Source: CAD feature listing. Evaluate the final solid. Frame: model axes, mm. A direction names the side the tool comes from. Coordinates: 2 decimals unless noted, no trailing zeros. Order: outer loops, then holes, each group sorted by start corner. A loop starts at its lowest first (then second) coordinate and runs counter-clockwise, first axis right, second up.
Item 1: Ray query, line 1 (X direction, y = 12.5, z = 18.5); line 2 (X direction, y = 3, z = 16); line 3 (Y direction, x = 19, z = 15.5) (3 decimals). Return the intervals inside material, ascending.
Item 2: Section C-C on x = -29.5. Return the cut outline in (y, z) (3 decimals).
Item 3: Section A-A on y = 11. Return the cut outline in (x, z).
Item 4: Section D-D on z = 21.25. Return the cut outline in (x, y) (3 decimals), then the cut area to 3 significant figures.
Item 5: Reachability of faces 1 (the flat face through (-35.306, 16, 13)), 2 (the flat face through (38.481, 18, 13)), 3 (the cylindrical face through (-51.128, 1.565, 19.875)) from +Z, -Z, +X, -X, +Y, -Y: full face, straight path, thin tool, end or side. Return the list, or none.
Item 6: Section B-B on z = 9.25. Return the cut outline in (x, y) (3 decimals), then the cut area to 3 significant figures.
Item 7: Contact query for flat-ended pins moving along their axis: P1, Ø8, axis at y = 15.5, z = 16, coming from the +X side; P2, Ø12.5, axis at x = -9.5, z = 8, coming from the -Y side; P3, Ø2, axis at y = 15, z = 15, coming from the -X side. Output: stop coordinate, or through.
from build123d import *

# Parameters (mm, degrees)
F1_DEPTH = 25.4
F2_R     = 3.175
F4_DEPTH = 32.386
F5_R     = 6.35


with BuildPart() as f1:
    # F0 (on Top) → F1 (new body)
    with BuildSketch(Plane.XY):
        Polygon((-35.306, 29.21), (0, 29.21), (35.306, 29.21), (35.306, 0), (63.881, 0), (63.881, 3.175), (38.481, 3.175), (38.481, 32.385), (0, 32.385), (-38.481, 32.385), (-38.481, 3.175), (-63.881, 3.175), (-63.881, 0), (-35.306, 0), align=None)
    extrude(amount=F1_DEPTH)

    # F2
    f2_edges = [f1.edges().sort_by_distance(p)[0] for p in [
        (-35.306, 0, 12.7),
        (35.306, 0, 12.7),
        (-38.481, 3.175, 12.7),
        (-38.481, 32.385, 12.7),
        (38.481, 32.385, 12.7),
        (38.481, 3.175, 12.7),
    ]]
    fillet(f2_edges, radius=F2_R)

    # F3 (on Front) → F4 (cut, through all)
    with BuildSketch(Plane.XZ):
        with BuildLine():
            ThreePointArc((-53.594, 7.8105), (-51.181, 5.3975), (-48.768, 7.8105))
            Line((-48.768, 7.8105), (-48.768, 17.4625))
            ThreePointArc((-48.768, 17.4625), (-51.181, 19.8755), (-53.594, 17.4625))
            Line((-53.594, 17.4625), (-53.594, 7.8105))
        make_face()
        with BuildLine():
            Line((48.768, 17.4625), (48.768, 7.8105))
            ThreePointArc((48.768, 7.8105), (51.181, 5.3975), (53.594, 7.8105))
            Line((53.594, 7.8105), (53.594, 17.4625))
            ThreePointArc((53.594, 17.4625), (51.181, 19.8755), (48.768, 17.4625))
        make_face()
    extrude(amount=-F4_DEPTH, mode=Mode.SUBTRACT)

    # F5
    f5_edges = [f1.edges().sort_by_distance(p)[0] for p in [
        (-63.881, 1.5875, 0),
        (-63.881, 1.5875, 25.4),
        (63.881, 1.5875, 25.4),
        (63.881, 1.5875, 0),
    ]]
    fillet(f5_edges, radius=F5_R)


solid = f1.part
Answer list:
1. line 1: x = -38.48 to -35.31, 35.31 to 38.48
1. line 2: x = -63.88 to -53.59, -48.77 to -35.31, 35.31 to 48.77, 53.59 to 63.88
1. line 3: y = 29.21 to 32.385
2. outline: (29.21, 0) - (32.385, 0) - (32.385, 25.4) - (29.21, 25.4) - close
3. outline: (-38.48, 0) - (-35.31, 0) - (-35.31, 25.4) - (-38.48, 25.4) - close; (35.31, 0) - (38.48, 0) - (38.48, 25.4) - (35.31, 25.4) - close
4. outline: (-63.488, 0) - (-38.481, 0) arc R3.175 ccw to (-35.306, 3.175) - (-35.306, 29.21) - (35.306, 29.21) - (35.306, 3.175) arc R3.175 ccw to (38.481, 0) - (63.488, 0) - (63.488, 3.175) - (41.656, 3.175) arc R3.175 cw to (38.481, 6.35) - (38.481, 29.21) arc R3.175 ccw to (35.306, 32.385) - (-35.306, 32.385) arc R3.175 ccw to (-38.481, 29.21) - (-38.481, 6.35) arc R3.175 cw to (-41.656, 3.175) - (-63.488, 3.175) - close
4. area: 584 mm2
5. face 1: +Z, -Z, -Y
5. face 2: +Z, -Z, +X, +Y
5. face 3: +Y, -Y
6. outline: (-63.881, 0) - (-53.594, 0) - (-53.594, 3.175) - (-63.881, 3.175) - close; (-48.768, 0) - (-38.481, 0) arc R3.175 ccw to (-35.306, 3.175) - (-35.306, 29.21) - (35.306, 29.21) - (35.306, 3.175) arc R3.175 ccw to (38.481, 0) - (48.768, 0) - (48.768, 3.175) - (41.656, 3.175) arc R3.175 cw to (38.481, 6.35) - (38.481, 29.21) arc R3.175 ccw to (35.306, 32.385) - (-35.306, 32.385) arc R3.175 ccw to (-38.481, 29.21) - (-38.481, 6.35) arc R3.175 cw to (-41.656, 3.175) - (-48.768, 3.175) - close; (53.594, 0) - (63.881, 0) - (63.881, 3.175) - (53.594, 3.175) - close
6. area: 556 mm2
7. P1: stops at x = 38.48
7. P2: stops at y = 29.21
7. P3: stops at x = -38.48
